```python
from build123d import *

# Parameters (mm, degrees)
SKETCH2_W           = 105
SKETCH2_H           = 25.118100445
BOSS_EXTRUDE2_DEPTH = 19
CUT_EXTRUDE13_DEPTH = 119
CUT_EXTRUDE15_DEPTH = 17
CUT_EXTRUDE17_DEPTH = 92
SKETCH8_R           = 4.186209529
CUT_EXTRUDE18_DEPTH = 92
BOSS_EXTRUDE3_DEPTH = 17
BOSS_EXTRUDE4_DEPTH = 17
SKETCH13_W          = 3.185616736
SKETCH13_H          = 3.062466768
BOSS_EXTRUDE6_DEPTH = 7.5
SKETCH14_W          = 3.051402249
SKETCH14_H          = 3.23810325
BOSS_EXTRUDE7_DEPTH = 7.5
FILLET1_R           = 5
FILLET2_R           = 5
FILLET5_R           = 8
FILLET6_R           = 8
SKETCH18_W          = 18
SKETCH18_H          = 12.3
CUT_EXTRUDE19_DEPTH = 15


with BuildPart() as part:
    # Sketch2 → Boss-Extrude2 (new body)
    with BuildSketch(Plane(origin=(0, 0, 0), x_dir=(1, 0, 0), z_dir=(0, 1, 0))):
        Polygon((-15, 76), (15, 76), (57.894125565, 58.485388954), (57.894125565, 27.051844623), (52.5, 18.118100445), (-52.5, 18.118100445), (-57.894125565, 27.051844623), (-57.894125565, 58.485388954), align=None)
        Polygon((52.5, -7), (-52.5, -7), (-52.5, -76), (0, -76), (15, -76), (52.5, -76), align=None)
        with Locations((0, 5.559050222)):
            Rectangle(SKETCH2_W, SKETCH2_H)
    extrude(amount=BOSS_EXTRUDE2_DEPTH)

    # Sketch4 → Cut-Extrude13 (cut)
    with BuildSketch(Plane(origin=(52.5, 0, 0), x_dir=(0, 0, -1), z_dir=(1, 0, 0))):
        Polygon((-76, 19), (-76, 9.5), (-7, 9.5), (18.118100445, 19), align=None)
    extrude(amount=-CUT_EXTRUDE13_DEPTH, mode=Mode.SUBTRACT)

    # Sketch5 → Cut-Extrude15 (cut)
    with BuildSketch(Plane(origin=(0, 19, 0), x_dir=(1, 0, 0), z_dir=(0, 1, 0))):
        Polygon((14.607411336, 74), (-14.607411336, 74), (-55.894125565, 57.141730213), (-55.894125565, 27.608811041), (-50.787885255, 19.151862072), (-50.5, 18.118100445), (50.5, 18.118100445), (50.787885255, 19.151862072), (55.894125565, 27.608811041), (55.894125565, 57.141730213), align=None)
    extrude(amount=-CUT_EXTRUDE15_DEPTH, mode=Mode.SUBTRACT)

    # Sketch7 → Cut-Extrude17 (cut)
    with BuildSketch(Plane(origin=(0, 0, -18.118100445), x_dir=(-1, 0, 0), z_dir=(0, 0, -1))):
        Polygon((50.5, 19), (50.5, 2), (11.545363278, 2), (-50.5, 2), (-50.5, 19), align=None)
    extrude(amount=-CUT_EXTRUDE17_DEPTH, mode=Mode.SUBTRACT)

    # Sketch8 → Cut-Extrude18 (cut)
    with BuildSketch(Plane(origin=(0, 0, -76), x_dir=(-1, 0, 0), z_dir=(0, 0, -1))):
        with Locations((0, 9.5)):
            Circle(SKETCH8_R)
    extrude(amount=-CUT_EXTRUDE18_DEPTH, mode=Mode.SUBTRACT)

    # Sketch11 → Boss-Extrude3 (add)
    with BuildSketch(Plane(origin=(0, 2, 0), x_dir=(1, 0, 0), z_dir=(0, 1, 0))):
        with BuildLine():
            Line((-51.347688624, 58.998140004), (-55.894125565, 57.141730213))
            Line((-55.894125565, 57.141730213), (-55.894125565, 52.230890552))
            ThreePointArc((-55.894125565, 52.230890552), (-53.106377647, 53.09885899), (-51.304073105, 55.395945406))
            Line((-51.304073105, 55.395945406), (-51.233975943, 55.592746134))
            ThreePointArc((-51.233975943, 55.592746134), (-50.986021462, 57.305621291), (-51.347688624, 58.998140004))
        make_face()
    extrude(amount=BOSS_EXTRUDE3_DEPTH)

    # Sketch12 → Boss-Extrude4 (add)
    with BuildSketch(Plane(origin=(0, 2, 0), x_dir=(1, 0, 0), z_dir=(0, 1, 0))):
        with BuildLine():
            Line((50.942379366, 58.29851863), (50.942379366, 57.141730213))
            ThreePointArc((50.942379366, 57.141730213), (52.392712249, 53.640316897), (55.894125565, 52.189984014))
            Line((55.894125565, 52.189984014), (55.894125565, 57.141730213))
            Line((55.894125565, 57.141730213), (51.18638565, 59.064003541))
            ThreePointArc((51.18638565, 59.064003541), (51.049240656, 58.686087709), (50.942379366, 58.29851863))
        make_face()
    extrude(amount=BOSS_EXTRUDE4_DEPTH)

    # Sketch13 → Boss-Extrude6 (add)
    with BuildSketch(Plane(origin=(0, 2, 0), x_dir=(1, 0, 0), z_dir=(0, 1, 0))):
        with Locations((48.907191632, -72.350666171)):
            Rectangle(SKETCH13_W, SKETCH13_H)
    extrude(amount=BOSS_EXTRUDE6_DEPTH)

    # Sketch14 → Boss-Extrude7 (add)
    with BuildSketch(Plane(origin=(0, 2, 0), x_dir=(1, 0, 0), z_dir=(0, 1, 0))):
        with Locations((-48.974298875, -72.26284793)):
            Rectangle(SKETCH14_W, SKETCH14_H)
    extrude(amount=BOSS_EXTRUDE7_DEPTH)

    # Fillet1
    fillet1_edges = [part.edges().sort_by_distance(p)[0] for p in [
        (-52.5, 4.75, 76),
    ]]
    fillet(fillet1_edges, radius=FILLET1_R)

    # Fillet2
    fillet2_edges = [part.edges().sort_by_distance(p)[0] for p in [
        (52.5, 4.75, 76),
    ]]
    fillet(fillet2_edges, radius=FILLET2_R)

    # Fillet5
    fillet5_edges = [part.edges().sort_by_distance(p)[0] for p in [
        (57.894125565, 9.5, -58.485388954),
    ]]
    fillet(fillet5_edges, radius=FILLET5_R)

    # Fillet6
    fillet6_edges = [part.edges().sort_by_distance(p)[0] for p in [
        (-57.894125565, 9.5, -58.485388954),
    ]]
    fillet(fillet6_edges, radius=FILLET6_R)

    # Sketch18 → Cut-Extrude19 (cut)
    with BuildSketch(Plane(origin=(-28.741404632, 0, -70.389083489), x_dir=(-0.925796249814304, 0, 0.37802288797078276), z_dir=(-0.37802288797078276, 0, -0.925796249814304))):
        with Locations((5.635958996, 9.5)):
            Rectangle(SKETCH18_W, SKETCH18_H)
    extrude(amount=-CUT_EXTRUDE19_DEPTH, mode=Mode.SUBTRACT)


solid = part.part
```
Input: part model. Units: mm. Frame: model coordinates. A direction names the side the tool comes from. Coordinates: 2 decimals unless noted, no trailing zeros. Loops run counter-clockwise (first coordinate to the right, second up) from the corner with the lowest first, then second, coordinate; pieces in that order, holes last. Notation, with made-up numbers: M -21.5,-23.75 L -11.5,-23.75 A12 cw -11.5,-8.75 Z; hole C 51,54.25 d6. An arc over 180 degrees is marked long. Use a Markdown table: item, result. Add a question column.
1) Line query: L1, parallel to Y at x = 0, z = -75; L2, parallel to X at y = 3, z = 61; L3, parallel to Y at x = 17.5, z = -49. Output: solid intervals per line, ascending. Write a range as from..to.
2) Set-up query: faces 1 (the cylindrical face through (56.57, 9.63, -57.52)), 2 (the flat face through (-52.5, 5, 26)), 3 (the flat face through (-50.5, 7, 16)). Return all of +Z, -Z, +X, -X, +Y, -Y with unobstructed straight access to the full face (end or side cutting, diameter ignored); none if empty.
3) Draft query along X for faces 4 (the cylindrical face through (52.354, 10.381, -53.679)), 5 (the flat face through (-53.377, 10.619, -23.44)), 6 (the cylindrical face through (-51.07, 4.82, 74.5)), 7 (the flat face through (55.235, 9.367, -22.648)). Return one class per face: +X half, -X half, draft (parallel to the pull), parting line (faces both ways), or undercut.
4) Section B-B, the plane z = 51. Return the cut outline in (x, y), plus the area to 3 significant figures.
5) Section D-D, the plane x = -38.5. Return the cut outline in (y, z).
6) Pin query (flat end, axial travel): P1, Ø6.5, axis at x = 0, y = 9.5, coming from the -Z side; P2, Ø1, axis at y = 6.5, z = 72.5, coming from the +X side; P3, Ø8, axis at x = 39, z = 21, coming from the +Y side; P4, Ø2.5, axis at x = -36, z = -67, coming from the -Y side. Return the tip coordinate at first contact, or that it passes through.
7) Section C-C, the plane x = 32. Return the cut outline in (y, z), plus the area to 3 significant figures.
8) Section A-A, the plane x = 0. Return the cut outline in (y, z).
Answer below:
| question | item | result |
|---|---|---|
| 1 | L1 | 0..5.31, 13.69..19 |
| 1 | L2 | -52.5..-50.5, 50.5..52.5 |
| 1 | L3 | 0..2 |
| 2 | face 1 | -Z, +X, +Y, -Y |
| 2 | face 2 | +Z, -X, +Y, -Y |
| 2 | face 3 | +Y |
| 3 | face 4 | undercut |
| 3 | face 5 | undercut |
| 3 | face 6 | -X half |
| 3 | face 7 | +X half |
| 4 | outline | M -52.5,0 L 52.5,0 L 52.5,9.5 L 50.5,9.5 L 50.5,2 L -50.5,2 L -50.5,9.5 L -52.5,9.5 Z |
| 4 | area | 240 mm2 |
| 5 | outline | M 0,-66.4 L 3.35,-66.4 L 3.35,-64.24 L 2,-64.24 L 2,73.88 L 9.5,73.88 L 9.5,76 L 0,76 Z; M 15.65,-66.4 L 19,-66.4 L 19,-64.24 L 15.65,-64.24 Z |
| 6 | P1 | z = 73.88 |
| 6 | P2 | x = 52.4 |
| 6 | P3 | y = 2 |
| 6 | P4 | y = 0 |
| 7 | outline | M 0,-69.06 L 19,-69.06 L 19,-66.9 L 2,-66.9 L 2,73.88 L 9.5,73.88 L 9.5,76 L 0,76 Z |
| 7 | area | 343 mm2 |
| 8 | outline | M 0,-76 L 5.31,-76 L 5.31,-74 L 2,-74 L 2,73.88 L 9.5,73.88 L 9.5,76 L 0,76 Z; M 13.69,-76 L 19,-76 L 19,-74 L 13.69,-74 Z |
